Here's how the part is built. I have some questions about the finished solid (model axes, mm). A direction names the side the tool comes from. Coordinates: 2 decimals unless noted, no trailing zeros. Order: outer loops, then holes, each group sorted by start corner. A loop starts at its lowest first (then second) coordinate and runs counter-clockwise, first axis right, second up. Notation, with made-up numbers: (-4, -40) - (26, -40) arc R12 ccw to (26, -33) - close; hole circle Ø11 at (29.5, 7). An arc over 180 degrees is marked (long way). Answer as CSV lines item,"result". Start each with the question number.
Q1. For faces 1 (the face through (-13, -10, 35.795)), 2 (the face through (-15.5, 4.88, 18.37)), which set-ups out of +Z, -Z, +X, -X, +Y, -Y let a thin tool reach every point of the face, with its end or its side?
Q2. For pin 1 Ø5 at (y, z) = (7, 16) entering from -X; pin 2 Ø20.5 at (x, y) = (0, 0) entering from +Z; pin 3 Ø4 at (x, z) = (-8, 10.5) entering from -Y; pin 4 Ø8 at (y, z) = (-2.5, 2.5) entering from +X, each with a flat end and sliding along its axis, tell me the tip position at first contact or that it passes through.
Q3. Suppose I cut it at C-C (z = -17). Please give me the cut outline in (x, y).
Q4. Suppose I cut it at D-D (z = 32). Please give me the cut outline in (x, y), then the cut area to 3 significant figures.
Q5. I need wall thicknesses on line 1 (Y direction, x = 0, z = 27); line 2 (Y direction, x = 0.5, z = -22); line 3 (X direction, y = -12.5, z = 2). Which ranges of each line are inside material? Lowest first, please.
Q6. Thinking about a two-plate mould opening in Y: for faces 3 (the face through (-11, -4, -32.157)), 4 (the face through (9.31, -7.14, -3.52)), 5 (the face through (-11.923, 3.755, -17.971)), which applies, released by +Y, released by -Y, zero draft, split by the parting line, or undercut?
Q7. Suppose I cut it at A-A (x = 0). Please give me the cut outline in (y, z), then the cut area to 3 significant figures.
from build123d import *

# Parameters (mm, degrees)
F0_W     = 17.25
F0_H     = 35.7945342632
F0_W_2   = 12.5
F0_H_2   = 27.9797699204
F3_T     = -1
F2_R     = 11.5
F4_DEPTH = 40


with BuildPart() as f1:
    # F0 (on Front) → F1 (revolve)
    with BuildSketch(Plane.XZ):
        with Locations((-8.625, 17.8972671316)):
            Rectangle(F0_W, F0_H)
        Polygon((0, -4.1769962882), (0, 0), (-17.25, 0), (-12.5, -4.1769962882), align=None)
        with Locations((-6.25, -18.1668812483)):
            Rectangle(F0_W_2, F0_H_2)
    revolve(axis=Axis((0, 0, 1.8188840273), (0, 0, -1)))

    # F3
    f3_openings = [f1.faces().sort_by_distance(p)[0] for p in [
        (0, 0, 35.794534),
    ]]
    offset(amount=F3_T, openings=f3_openings, kind=Kind.INTERSECTION)

    # F2 (on face) → F4 (cut)
    with BuildSketch(Plane(origin=(0, 0, -32.1567662085), x_dir=(1, 0, 0), z_dir=(0, 0, -1))):
        Circle(F2_R)
    extrude(amount=-F4_DEPTH, mode=Mode.SUBTRACT)


solid = f1.part
Here are the results:
1,face 1,"+Z, +X, -X, +Y, -Y"
1,face 2,"+Z"
2,pin 1,"stops at x = -16.65"
2,pin 2,"passes through"
2,pin 3,"stops at y = -16.17"
2,pin 4,"stops at x = 17.25"
3,outline,"circle Ø25 at (0, 0); hole circle Ø23 at (0, 0)"
4,outline,"circle Ø34.5 at (0, 0); hole circle Ø32.5 at (0, 0)"
4,area,"105 mm²"
5,line 1,"y = -17.25 to -16.25, 16.25 to 17.25"
5,line 2,"y = -12.49 to -11.49, 11.49 to 12.49"
5,line 3,"x = -11.89 to -10.38, 10.38 to 11.89"
6,face 3,"zero draft"
6,face 4,"undercut"
6,face 5,"split by the parting line"
7,outline,"(-17.25, 0) - (-12.5, -4.18) - (-12.5, -32.16) - (-11.5, -32.16) - (-11.5, -3.72) - (-16.25, 0.45) - (-16.25, 35.79) - (-17.25, 35.79) - close; (11.5, -32.16) - (12.5, -32.16) - (12.5, -4.18) - (17.25, 0) - (17.25, 35.79) - (16.25, 35.79) - (16.25, 0.45) - (11.5, -3.72) - close"
7,area,"140 mm²"
